Source: CAD feature listing. Evaluate the final solid. Frame: model axes, mm. Give positions to 0.01 mm unless a question says otherwise; leave off trailing zeros. Write each loop counter-clockwise with the first axis right and the second up, starting at its lowest first coordinate (ties: lowest second). Pieces come first, ordered by that corner, then holes. Notation, with made-up numbers: M 63,86.5 L 107,86.5 A19 cw 107,99.5 Z; hole C 83.25,87.5 d7. An arc over 180 degrees is marked long. Use CSV: the item, a comma, the result in double quotes. Start each with the question number.
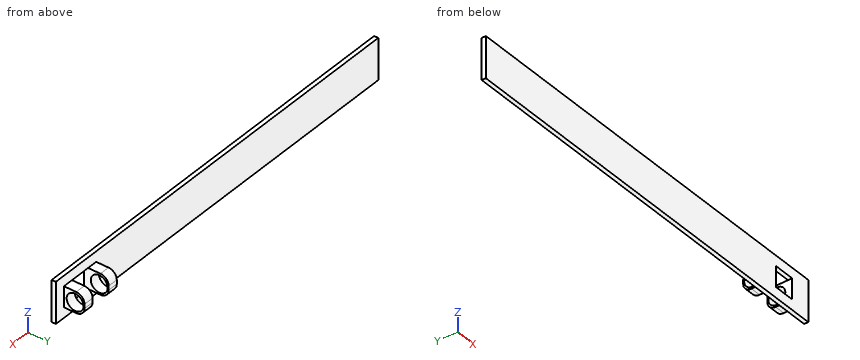
from build123d import *

# Parameters (mm, degrees)
SKETCH1_W             = 2.5
SKETCH1_H             = 5
BOSS_EXTRUDE1_DEPTH   = 5
BOSS_EXTRUDE1_2_DEPTH = 5
SKETCH1_3_W           = 100
SKETCH1_3_H           = 10
SKETCH1_3_W_2         = 10
SKETCH1_3_H_2         = 5
BOSS_EXTRUDE2_DEPTH   = 1
SKETCH1_4_W           = 2.5
SKETCH1_4_H           = 5
BOSS_EXTRUDE3_DEPTH   = 1
SKETCH2_R             = 2.05
CUT_EXTRUDE1_DEPTH    = 98.5
FILLET1_R             = 2


with BuildPart() as part:
    # Sketch1 → Boss-Extrude1 (new body)
    with BuildSketch(Plane(origin=(0, 0, 0), x_dir=(1, 0, 0), z_dir=(0, 1, 0))):
        with Locations((88.75, 5)):
            Rectangle(SKETCH1_W, SKETCH1_H)
    extrude(amount=BOSS_EXTRUDE1_DEPTH)



with BuildPart() as body_2:
    # Sketch1 → Boss-Extrude1 2 (new body)
    with BuildSketch(Plane(origin=(0, 0, 0), x_dir=(1, 0, 0), z_dir=(0, 1, 0))):
        with Locations((96.25, 5)):
            Rectangle(SKETCH1_W, SKETCH1_H)
    extrude(amount=BOSS_EXTRUDE1_2_DEPTH)


with BuildPart() as body_3:
    # Sketch1_3 → Boss-Extrude2 (new body)
    with BuildSketch(Plane(origin=(0, 0, 0), x_dir=(1, 0, 0), z_dir=(0, 1, 0))):
        with Locations((50, 5)):
            Rectangle(SKETCH1_3_W, SKETCH1_3_H)
        with Locations((92.5, 5)):
            Rectangle(SKETCH1_3_W_2, SKETCH1_3_H_2, mode=Mode.SUBTRACT)
    extrude(amount=-BOSS_EXTRUDE2_DEPTH)


with BuildPart() as part_1:
    add(part.part)

    add(body_2.part)  # Boss-Extrude3 merges body 2

    add(body_3.part)  # Boss-Extrude3 merges body 3
    # Sketch1_4 → Boss-Extrude3 (add)
    with BuildSketch(Plane(origin=(0, 0, 0), x_dir=(1, 0, 0), z_dir=(0, 1, 0))):
        with Locations((88.75, 5)):
            Rectangle(SKETCH1_4_W, SKETCH1_4_H)
        with Locations((96.25, 5)):
            Rectangle(SKETCH1_4_W, SKETCH1_4_H)
    extrude(amount=-BOSS_EXTRUDE3_DEPTH)

    # Sketch2 → Cut-Extrude1 (cut, through all)
    with BuildSketch(Plane(origin=(97.5, 0, 0), x_dir=(0, 0, -1), z_dir=(1, 0, 0))):
        with Locations((5.065113553, 2.710102322)):
            Circle(SKETCH2_R)
    extrude(amount=-CUT_EXTRUDE1_DEPTH, mode=Mode.SUBTRACT)

    # Fillet1
    fillet1_edges = [part_1.edges().sort_by_distance(p)[0] for p in [
        (88.75, 5, -7.5),
        (88.75, 5, -2.5),
        (96.25, 5, -7.5),
        (96.25, 5, -2.5),
    ]]
    fillet(fillet1_edges, radius=FILLET1_R)


solid = part_1.part
1. Section B-B on x = 37. Return loops of the section in (y, z), then the cut area to 3 significant figures.
2. Section A-A on z = -8.75. Return loops of the section in (x, y), then the cut area to 3 significant figures.
3. Line query: probe 1 along X at (y, z) = (-0.2, -3.25); probe 2 along X at (y, z) = (0.7, -4.5); probe 3 along Y at (x, z) = (36, -9.5). Output: solid intervals per line, ascending.
4. First-contact query: pin 1 (2 mm diameter, centred on x = 49, z = -4.5, fed in from +Y); pin 2 (0.8 mm diameter, centred on x = 92, y = -0.5, fed in from +Z); pin 3 (3.5 mm diameter, centred on y = 2.71, z = -5.07, fed in from -X); pin 4 (0.8 mm diameter, centred on x = 89, y = 1.5, fed in from +Z). Flat tips, straight axial feed; report the tip coordinate or a pass-through.
Resolved:
1,outline,"M -1,-10 L 0,-10 L 0,0 L -1,0 Z"
1,area,"10.0 mm2"
2,outline,"M 0,-1 L 100,-1 L 100,0 L 0,0 Z"
2,area,"100 mm2"
3,probe 1,"x = 0 to 90, 95 to 100"
3,probe 2,"x = 87.5 to 90, 95 to 97.5"
3,probe 3,"y = -1 to 0"
4,pin 1,"stops at y = 0"
4,pin 2,"stops at z = 0"
4,pin 3,"passes through"
4,pin 4,"stops at z = -2.5"
